from build123d import *

# Parameters (mm, degrees)
F3_D    = 10
F5_SIZE = 1
F6_D    = 3.3


with BuildPart() as f1:
    # F0 (on Right) → F1 (revolve)
    with BuildSketch(Plane.YZ):
        Polygon((-13.6, 0), (0, 0), (0, 30), (-13.6, 26.875), align=None)
    revolve(axis=Axis((0, -6.8, 0), (0, -1, 0)))

    # F3 (through all)
    with Locations(Plane(origin=(0, 0, 0), x_dir=(-1, 0, 0), z_dir=(0, 1, 0))):
        with Locations((0, 0)):
            Hole(F3_D / 2)

    # F5
    f5_edges = [f1.edges().sort_by_distance(p)[0] for p in [
        (0, -13.6, -26.875),
    ]]
    chamfer(f5_edges, length=F5_SIZE)

    # F6 (through all)
    with Locations(Plane.XZ.offset(13.6)):
        with Locations((0, 21.8), (21.8, 0), (0, -21.8), (-21.8, 0)):
            Hole(F6_D / 2)


solid = f1.part
Design review of the part built by this model. Coordinates are the model's own, in mm. Round coordinates to 2 decimals unless told otherwise and drop trailing zeros. Loops run counter-clockwise (first coordinate to the right, second up) from the corner with the lowest first, then second, coordinate; pieces in that order, holes last. Notation, with made-up numbers: (-14, 0.25) - (25, 0.25) arc R30 cw to (25, 37.25) - close; hole circle Ø6 at (85, -11). An arc over 180 degrees is marked (long way). One line per question, with ' | ' between items.
1. Clearance check with flat-ended pins moving along their axes: P1, Ø5.5, axis at x = 0, z = -21.8, coming from the -Y side; P2, Ø8, axis at x = 5.5, y = -8.5, coming from the -Z side; P3, Ø5, axis at y = -8.5, z = 6.5, coming from the +X side; P4, Ø6, axis at y = -11, z = 19, coming from the +X side. State where each tip first meets the part, or that it passes through.
Results are:
P1: stops at y = -13.6 | P2: stops at z = -28.63 | P3: stops at x = 28.06 | P4: stops at x = 22.49
2. Draft analysis for pull direction Z (two halves, no side actions). For faces 1 (the face through (-0.89, -6.7, 23.19)), 2 (the face through (5.4, -13.6, -0.4)), 3 (the face through (-27.01, -12.01, -3.55)), state which applies: released by +Z, released by -Z, zero draft, split by the parting line, or undercut.
Results are:
face 1: undercut | face 2: zero draft | face 3: split by the parting line
3. For L1, parallel to Z at x = 0, y = -9; L2, parallel to Z at x = -1.5, y = -7.5; L3, parallel to X at y = -7.5, z = -4, list the stretches that pass through material, from the lowest coordinate up. Write a range as [from, to].
Results are:
L1: z = [-27.93, -23.45], [-20.15, -5], [5, 20.15], [23.45, 27.93] | L2: z = [-28.24, -22.49], [-21.11, -4.77], [4.77, 21.11], [22.49, 28.24] | L3: x = [-27.99, -3], [3, 27.99]
4. We need section C-C, the plane y = -10.25. State the section outline as (x, z) points, and give its area (3 significant figures).
Results are:
outline: circle Ø55.29 at (0, 0); hole circle Ø3.3 at (-21.8, 0); hole circle Ø10 at (0, 0); hole circle Ø3.3 at (0, -21.8); hole circle Ø3.3 at (0, 21.8); hole circle Ø3.3 at (21.8, 0) | area: 2,290 mm²
5. We need section B-B, the plane x = 0. State the section outline as (y, z) points (3 decimals).
Results are:
outline: (-13.6, -25.875) - (-12.625, -27.099) - (0, -30) - (0, -23.45) - (-13.6, -23.45) - close; (-13.6, -20.15) - (0, -20.15) - (0, -5) - (-13.6, -5) - close; (-13.6, 5) - (0, 5) - (0, 20.15) - (-13.6, 20.15) - close; (-13.6, 23.45) - (0, 23.45) - (0, 30) - (-12.625, 27.099) - (-13.6, 25.875) - close
6. We need section A-A, the plane z = 0. State the section outline as (x, y) points (3 decimals).
Results are:
outline: (-30, 0) - (-27.099, -12.625) - (-25.875, -13.6) - (-23.45, -13.6) - (-23.45, 0) - close; (-20.15, -13.6) - (-5, -13.6) - (-5, 0) - (-20.15, 0) - close; (5, -13.6) - (20.15, -13.6) - (20.15, 0) - (5, 0) - close; (23.45, -13.6) - (25.875, -13.6) - (27.099, -12.625) - (30, 0) - (23.45, 0) - close
